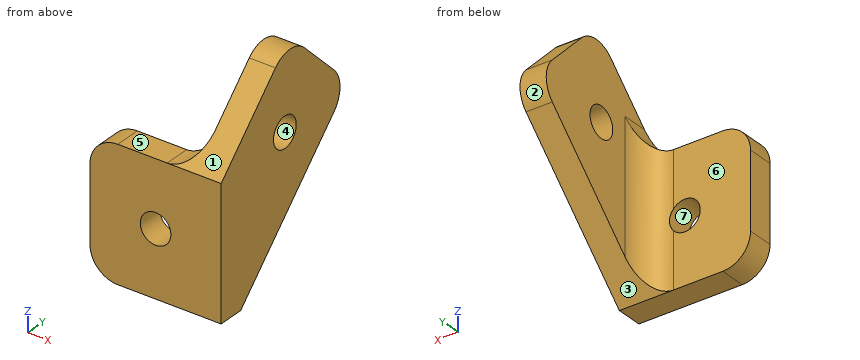
Autodesk Inventor part; units mm, degrees
ref_plane "YZ Plane" through (0, 0, 0) normal (1, 0, 0) x (0, 1, 0)
ref_plane "XZ Plane" through (0, 0, 0) normal (0, 1, 0) x (-1, 0, 0)
ref_plane "XY Plane" through (0, 0, 0) normal (0, 0, 1) x (1, 0, 0)
sketch "Sketch1" plane through (0, 0, 0) normal (0, 1, 0) x (-1, 0, 0)
  line L0 (0, 0) -> (15, 0)
  line L1 (15, 0) -> (15, -15)
  line L2 (15, -15) -> (0, -15)
  line L3 (0, -15) -> (0, 0)
  circle A0 centre (7.5, -7.5) radius 1.75
  dimension "d0" = 15
  dimension "d1" = 15
  dimension "d2" = 3.5
extrude "Extrusion1" add sketch "Sketch1" along normal blind 3
sketch "Sketch2" plane through (0, 0, 0) normal (1, 0, 0) x (0, 0, -1)
  line L0 (15, 0) -> (0, 0)
  line L1 (0, 0) -> (-10.6066, 10.6066)
  line L2 (0, 0) -> (15, 0) construction
  line L3 (15, 0) -> (40.6066, 0) construction
  line L4 (-3.1066, 18.1066) -> (-10.6066, 10.6066)
  line L5 (15, 3) -> (0, 3)
  line L6 (15, 3) -> (-1.6066, 19.6066)
  line L7 (15, 3) -> (38.4853, 3) construction
  line L8 (-1.6066, 19.6066) -> (-3.1066, 18.1066)
  line L9 (-1.6066, 19.6066) -> (-10.6066, 10.6066) construction
  line L10 (-6.1066, 15.1066) -> (7.5, 1.5) construction
  circle A0 centre (-0.8033, 9.8033) radius 1.75
  line L11 (15, 3) -> (15, 0)
  line L12 (0, 0) -> (15, 0)
  line L13 (15, 3) -> (-1.6066, 19.6066)
  line L14 (-1.6066, 19.6066) -> (-10.6066, 10.6066)
  line L15 (-10.6066, 10.6066) -> (0, 0)
  dimension "d5" = 15
  dimension "d6" = 135
  dimension "d10" = 135
  dimension "d12" = 3.5
  dimension "d13" = 7.5
extrude "Extrusion3" add sketch "Sketch2" against normal blind 3
fillet "Fillet1" radius 3.175 4 edges at (-15, 1.5, -15) (-15, 1.5, 0) (-1.5, 19.6066, 1.6066) (-1.5, 10.6066, 10.6066)
fillet "Fillet2" radius 3.175 2 edges at (-3, 3, -7.5) (-3, 1.5, 0)
properties part number "45 degree inside angle bracket_3DPrint"
Read the model definition and answer for the solid it produces. Units are mm, in the model's axes. Face numbers are marked on the shaded views. A direction names the side the tool comes from. Round coordinates to 2 decimals unless told otherwise and drop trailing zeros. Write each loop counter-clockwise with the first axis right and the second up, starting at its lowest first coordinate (ties: lowest second). Pieces come first, ordered by that corner, then holes. Notation, with made-up numbers: (63, 31.25) -> (67, 31.25) arc R38 ccw to (67, 70.25) -> close; hole circle Ø6 at (-17.75, 56.5). An arc over 180 degrees is marked (long way). Answer in a Markdown table with one row per item. Add a question column.
1) Which of the six approach directions +Z, -Z, +X, -X, +Y, -Y give full straight-line access (tool end or side, diameter ignored) to the marked faces 5, 6 and 7?
2) Determine the mould class of the marked faces 1, 2, 3 and 4 for opening direction Z: pulls with the +Z half, pulls with the -Z half, needs draft (parallel to the pull), parting line crosses it, or undercut.
3) Consider line 1 (Z direction, x = -7.5, y = 1.9); line 2 (Y direction, x = -9.5, z = -9.25). Determine where each line is inside the solid, lowest interval first.
4) Given P1, Ø2, axis at x = -1.5, y = 10, coming from the -Z side; P2, Ø4.5, axis at x = -8.5, z = -11, coming from the +Y side; P3, Ø5.5, axis at y = 9.8, z = 0.8, coming from the +X side; P4, Ø1, axis at x = -2, z = -5.5, coming from the +Y side, each flat-ended and moving along its own axis, determine where each tip first touches the part or whether it passes through.
5) Find section C-C, the plane y = 9.25. Determine the outline of the cut face in (x, z), and give its area (3 significant figures).
6) Find section D-D, the plane x = -0.75. Determine the outline of the cut face in (y, z) (3 decimals).
7) Find section A-A, the plane z = -7.5. Determine the outline of the cut face in (x, y) (3 decimals), and give its area (3 significant figures).
8) Find section B-B, the plane x = -7.5. Determine the outline of the cut face in (y, z).
Findings below:
| question | item | result |
|---|---|---|
| 1 | face 5 | +Z, -X, +Y, -Y |
| 1 | face 6 | +Z, -Z, -X, +Y |
| 1 | face 7 | +Y, -Y |
| 2 | face 1 | pulls with the +Z half |
| 2 | face 2 | parting line crosses it |
| 2 | face 3 | pulls with the -Z half |
| 2 | face 4 | undercut |
| 3 | line 1 | -15 to -9.25, -5.75 to 0 |
| 3 | line 2 | 0 to 3 |
| 4 | P1 | z = -9 |
| 4 | P2 | y = 3 |
| 4 | P3 | x = 0 |
| 4 | P4 | y = 13 |
| 5 | outline | (-3, -8.75) -> (0, -8.75) -> (0, -0.86) -> (-3, -0.86) -> close; (-3, 2.46) -> (0, 2.46) -> (0, 8.99) -> (-3, 8.99) -> close |
| 5 | area | 43.2 mm² |
| 6 | outline | (0, -15) -> (3, -15) -> (17.362, -0.638) arc R3.175 ccw to (17.362, 3.852) -> (12.852, 8.362) arc R3.175 ccw to (8.362, 8.362) -> (0, 0) -> close; hole circle Ø3.5 at (9.803, 0.803) |
| 7 | outline | (-15, 0) -> (-9.25, 0) -> (-9.25, 3) -> (-15, 3) -> close; (-5.75, 0) -> (0, 0) -> (0, 10.5) -> (-3, 10.5) -> (-3, 6.175) arc R3.175 cw to (-5.75, 3.029) -> close |
| 7 | area | 59.2 mm² |
| 8 | outline | (0, -15) -> (3, -15) -> (3, -9.25) -> (0, -9.25) -> close; (0, -5.75) -> (3, -5.75) -> (3, 0) -> (0, 0) -> close |
